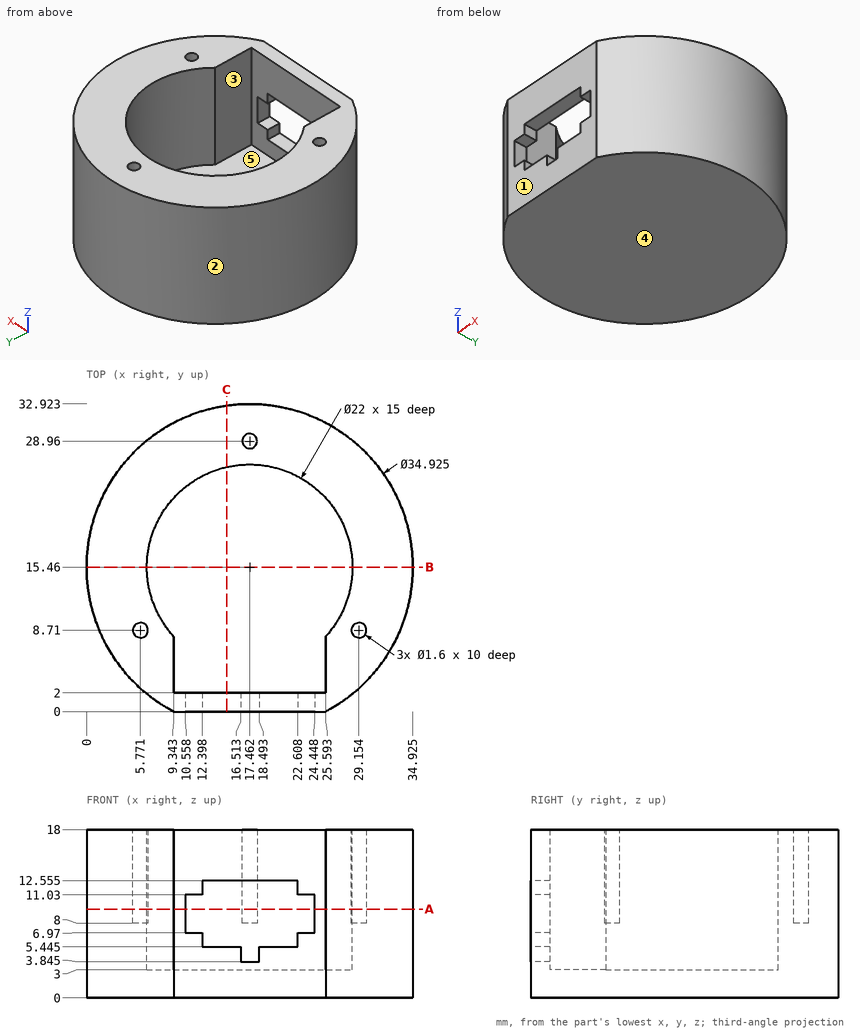
Source: three-view drawing plus pictorial views. Frame: mm from the lowest corner of the part. A direction names the side the tool comes from. Coordinates: 2 decimals unless noted, no trailing zeros. Order: outer loops, then holes, each group sorted by start corner. A loop starts at its lowest first (then second) coordinate and runs counter-clockwise, first axis right, second up. Notation, with made-up numbers: M -17.75,-32.75 L -2.75,-32.75 A21 cw -2.75,1.25 Z; hole C 43,-23 d5. An arc over 180 degrees is marked long. One line per question, with ' | ' between items.
Item 1: Draft query along X for the marked faces 1, 2 and 3. Return one class per face: released by +X, released by -X, zero draft, split by the parting line, or undercut.
Geometry results:
face 1: zero draft | face 2: split by the parting line | face 3: undercut
Item 2: Reachability of the marked faces 4 and 5 from +Z, -Z, +X, -X, +Y, -Y: full face, straight path, thin tool, end or side. Return the list, or none.
Geometry results:
face 4: -Z, +X, -X, +Y, -Y | face 5: +Z
Item 3: Ray query, line 1 along Z through (x, y) = (17.5, 6); line 2 along X through (y, z) = (7, 7.25) (1 decimal); line 3 along X through (y, z) = (10.5, 14.75) (1 decimal). Return the intervals inside material, ascending.
Geometry results:
line 1: z = 0 to 3 | line 2: x = 2.2 to 9.3, 25.6 to 32.7 | line 3: x = 0.7 to 7.6, 27.3 to 34.2
Item 4: Section B-B (y = 15.46). Output: boundary loops of the cut face in (x, z) (1 decimal).
Geometry results:
outline: M 0,0 L 34.9,0 L 34.9,18 L 28.5,18 L 28.5,3 L 6.5,3 L 6.5,18 L 0,18 Z
Item 5: Pin query (flat end, axial travel): pin 1 (8 mm diameter, centred on y = 24, z = 16, fed in from -X); pin 2 (2 mm diameter, centred on y = 1.5, z = 8, fed in from +X) (1 decimal); pin 3 (5 mm diameter, centred on x = 10, z = 4, fed in from +Y). Return the tip coordinate at first contact, or that it passes through.
Geometry results:
pin 1: stops at x = 0.6 | pin 2: stops at x = 29.2 | pin 3: stops at y = 32.2
Item 6: Section C-C (x = 15). Output: boundary loops of the cut face in (y, z) (1 decimal).
Geometry results:
outline: M 0,0 L 32.7,0 L 32.7,18 L 26.2,18 L 26.2,3 L 2,3 L 2,5.4 L 0,5.4 Z; M 0,12.6 L 2,12.6 L 2,18 L 0,18 Z
Item 7: Section A-A (z = 9.5). Give the number of separate pieces and of enclosed holes in the cut face, then the cut area to 3 significant figures.
Geometry results:
separate pieces: 1 | enclosed holes: 3 | area: 464 mm^2
